Input: part model. Units: mm. Frame: model coordinates. A direction names the side the tool comes from. Give positions to 0.01 mm unless a question says otherwise; leave off trailing zeros. Write each loop counter-clockwise with the first axis right and the second up, starting at its lowest first coordinate (ties: lowest second). Pieces come first, ordered by that corner, then holes. Notation, with made-up numbers: M 78,29 L 108,29 A32 ccw 108,62 Z; hole C -27.75,83 d11. An arc over 180 degrees is marked long. Use CSV: the item, a comma, the result in double quotes. Start each with the question number.
from build123d import *

# Parameters (mm, degrees)
SKETCH1_R           = 3.903170007
SKETCH1_R_2         = 4.085841865
BOSS_EXTRUDE1_DEPTH = 5


with BuildPart() as part:
    # Sketch1 → Boss-Extrude1 (new, symmetric)
    with BuildSketch(Plane.XY):
        Polygon((24.873664066, 25), (-25, 25), (-35, 15), (-35, -24.873664066), (-25.252671867, -24.873664066), (-25.252671867, -15.08356524), (-15.252671867, -15.08356524), (-15.252671867, -15.209901174), (-15, -15.209901174), (-15, -24.873664066), (14.747328133, -24.873664066), (14.747328133, -11.089222254), (24.747328133, -11.089222254), (24.747328133, -11.215558187), (25, -11.215558187), (25, -24.873664066), (34.747328133, -24.873664066), (34.747328133, 15.126335934), align=None)
        Polygon((15, -10), (-15, -10), (-15, 0.964343272), (-8.398565663, 0.964343272), (-8.398565663, -4.035656728), (8.398565663, -4.035656728), (8.398565663, 0.964343272), (15, 0.964343272), align=None, mode=Mode.SUBTRACT)
        with Locations((-25, 15)):
            Circle(SKETCH1_R, mode=Mode.SUBTRACT)
        with Locations((25, 15)):
            Circle(SKETCH1_R_2, mode=Mode.SUBTRACT)
    extrude(amount=BOSS_EXTRUDE1_DEPTH, both=True)


solid = part.part
Q1. Pull-direction query (X, two-part tool) for faces 4 (the cylindrical face through (20.92, 15.18, -0.07)), 5 (the flat face through (-35, -5, 0)), 6 (the flat face through (-1, 0, 5)); classes: released by +X, released by -X, zero draft, split by the parting line, or undercut.
Q2. Section C-C, the plane y = -5.5. Return the cut outline in (x, z), and give its area (3 significant figures).
Q3. Section A-A, the plane y = -22. Return the cut outline in (x, z).
Q4. First-contact query: pin 1 Ø6.5 at (x, y) = (25, 15) entering from +Z. Flat tip, straight axial feed; report the tip coordinate or a pass-through.
Q5. Section B-B, the plane x = -12. Return the cut outline in (y, z), and give its area (3 significant figures).
Q6. Material intervals for L1, parallel to Y at x = 4, z = -4.5; L2, parallel to Y at x = -14, z = -1.25; L3, parallel to X at y = 0, z = -3.75, sorted ascending. Write a range as [from, to].
Q7. Set-up query: faces 1 (the flat face through (0, -4.036, 0)), 2 (the flat face through (0, 25, 0)), 3 (the flat face through (-20, -15.084, 0)). Return all of +Z, -Z, +X, -X, +Y, -Y with unobstructed straight access to the full face (end or side cutting, diameter ignored); none if empty.
Q8. Section D-D, the plane z = -3. Return the cut outline in (x, y), and give its area (3 significant figures).
Check result:
1,face 4,"undercut"
1,face 5,"released by -X"
1,face 6,"zero draft"
2,outline,"M -35,-5 L -15,-5 L -15,5 L -35,5 Z; M 15,-5 L 34.75,-5 L 34.75,5 L 15,5 Z"
2,area,"397 mm²"
3,outline,"M -35,-5 L -25.25,-5 L -25.25,5 L -35,5 Z; M -15,-5 L 14.75,-5 L 14.75,5 L -15,5 Z; M 25,-5 L 34.75,-5 L 34.75,5 L 25,5 Z"
4,pin 1,"passes through"
5,outline,"M -24.87,-5 L -10,-5 L -10,5 L -24.87,5 Z; M 0.96,-5 L 25,-5 L 25,5 L 0.96,5 Z"
5,area,"389 mm²"
6,L1,"y = [-24.87, -10], [-4.04, 25]"
6,L2,"y = [-24.87, -10], [0.96, 25]"
6,L3,"x = [-35, -15], [-8.4, 8.4], [15, 34.75]"
7,face 1,"+Z, -Z"
7,face 2,"+Z, -Z, +X, -X, +Y"
7,face 3,"+Z, -Z, -Y"
8,outline,"M -35,-24.87 L -25.25,-24.87 L -25.25,-15.08 L -15.25,-15.08 L -15.25,-15.21 L -15,-15.21 L -15,-24.87 L 14.75,-24.87 L 14.75,-11.09 L 24.75,-11.09 L 24.75,-11.22 L 25,-11.22 L 25,-24.87 L 34.75,-24.87 L 34.75,15.13 L 24.87,25 L -25,25 L -35,15 Z; hole C -25,15 d7.81; hole M -15,-10 L 15,-10 L 15,0.96 L 8.4,0.96 L 8.4,-4.04 L -8.4,-4.04 L -8.4,0.96 L -15,0.96 Z; hole C 25,15 d8.17"
8,area,"2,790 mm²"
